from build123d import *

# Parameters (mm, degrees)
EXTRUDE_1_DEPTH     = 12
SKETCH_3_R          = 11
CUT_EXTRUDE_1_DEPTH = 111
SKETCH_4_R          = 12.5
CUT_EXTRUDE_2_DEPTH = 124.693168769
SKETCH_5_W          = 8
SKETCH_5_H          = 15.8
CUT_EXTRUDE_3_DEPTH = 124.693168769
SKETCH_6_R          = 3.4
CUT_EXTRUDE_4_DEPTH = 13
SKETCH_7_R          = 2.5
CUT_EXTRUDE_5_DEPTH = 10


with BuildPart() as part:
    # 草图1 → 旋转1 (revolve)
    with BuildSketch(Plane(origin=(0, 0, 0), x_dir=(1, 0, 0), z_dir=(0, 1, 0)), mode=Mode.PRIVATE) as revolve_1_sk:
        Polygon((0, 0), (25, 0), (25, -45), (40, -45), (40, -55), (0, -55), align=None)
    revolve(revolve_1_sk.sketch.rotate(Axis((0, 0, 0), (0, 0, 1)), 180), axis=Axis((0, 0, 0), (0, 0, 1)))

    # 草图2 → 凸台-拉伸1 (add)
    with BuildSketch(Plane(origin=(24, 0, 0), x_dir=(0, 0, -1), z_dir=(1, 0, 0))):
        with BuildLine():
            Line((-45, -20), (-90, -20))
            ThreePointArc((-90, -20), (-110, 0), (-90, 20))
            Line((-90, 20), (-45, 20))
            Line((-45, 20), (-45, -20))
        make_face()
    extrude_1 = extrude(amount=EXTRUDE_1_DEPTH)

    # 镜向1: 凸台-拉伸1 across plane
    add(extrude_1.mirror(Plane(origin=(0, 0, 0), x_dir=(0, 0, 1), z_dir=(1, 0, 0))))

    # 草图3 → 切除-拉伸1 (cut, symmetric)
    with BuildSketch(Plane(origin=(0, 0, 0), x_dir=(0, 0, -1), z_dir=(1, 0, 0))):
        with Locations((-90, 0)):
            Circle(SKETCH_3_R)
    extrude(amount=CUT_EXTRUDE_1_DEPTH, both=True, mode=Mode.SUBTRACT)

    # 草图4 → 切除-拉伸2 (cut, through all)
    with BuildSketch(Plane.XY):
        with Locations(Location((0, 0, 0), (0, 0, 180))):
            Circle(SKETCH_4_R)
    extrude(amount=CUT_EXTRUDE_2_DEPTH, mode=Mode.SUBTRACT)

    # 草图5 → 切除-拉伸3 (cut, through all)
    with BuildSketch(Plane.XY):
        with Locations((0, 7.9)):
            Rectangle(SKETCH_5_W, SKETCH_5_H)
    extrude(amount=CUT_EXTRUDE_3_DEPTH, mode=Mode.SUBTRACT)

    # 草图6 → 切除-拉伸4 (cut)
    with BuildSketch(Plane(origin=(0, 25, 0), x_dir=(1, 0, 0), z_dir=(0, 1, 0))):
        with Locations(Location((0, -20, 0), (0, 0, 270))):
            Circle(SKETCH_6_R)
    extrude(amount=-CUT_EXTRUDE_4_DEPTH, mode=Mode.SUBTRACT)

    # 草图7 → 切除-拉伸5 (cut)
    with BuildSketch(Plane(origin=(36, 0, 0), x_dir=(0, 0, -1), z_dir=(1, 0, 0))):
        with Locations((-90, 14.5)):
            Circle(SKETCH_7_R)
        with Locations((-90, -14.5)):
            Circle(SKETCH_7_R)
    cut_extrude_5 = extrude(amount=-CUT_EXTRUDE_5_DEPTH, mode=Mode.SUBTRACT)

    # 镜向2: 切除-拉伸5 across plane
    add(cut_extrude_5.mirror(Plane(origin=(0, 0, 0), x_dir=(0, 0, 1), z_dir=(1, 0, 0))), mode=Mode.SUBTRACT)


solid = part.part
Build history of the part. All positions in model axes, mm. A direction names the side the tool comes from. Give positions to 0.01 mm unless a question says otherwise; leave off trailing zeros. Order: outer loops, then holes, each group sorted by start corner. A loop starts at its lowest first (then second) coordinate and runs counter-clockwise, first axis right, second up. Notation, with made-up numbers: M 17,57.25 L 30,57.25 A17 ccw 30,87.25 Z; hole C -12,-8.75 d2. An arc over 180 degrees is marked long. Put each result on its own line as item: value.
Item 1: 3-axis set-ups, long thin cutter, end or side, ignore diameter. For faces 1 (the flat face through (-26, 15, 90)), 2 (the flat face through (-18.34, 17.22, 45)), 3 (the flat face through (24, 0, 76)): which of +Z, -Z, +X, -X, +Y, -Y reach the whole face in a straight line?
From the geometry:
face 1: -X
face 2: -Z
face 3: +Z, +Y, -Y
Item 2: Two-plate mould, pull along Z, no slides. Class faces 4 (the flat face through (-36, 0, 77)), 5 (the flat face through (-38, 0, 55)), 6 (the cylindrical face through (-30, 0, 101)): +Z half, -Z half, draft (parallel to the pull), parting line (faces both ways), or undercut.
From the geometry:
face 4: draft
face 5: +Z half
face 6: undercut
Item 3: Flat gauge pins, fed straight in: pin 1 Ø4.5 at (y, z) = (14.5, 90) entering from +X; pin 2 Ø4 at (x, z) = (-1, 34) entering from -Y; pin 3 Ø5.5 at (x, z) = (0, 20) entering from +Y. Where does each tip first touch, or does it go through?
From the geometry:
pin 1: stops at x = 26
pin 2: stops at y = -25
pin 3: stops at y = -12.19
Item 4: Probe line 1 (Y direction, x = -31.75, z = 90); line 2 (X direction, y = -0.5, z = 64); line 3 (Z direction, x = 0, y = 18.5). List the from-to ranges inside material, lowest first. Write a range as [from, to].
From the geometry:
line 1: y = [-20, -17], [-12, -11], [11, 12], [17, 20]
line 2: x = [-36, -24], [24, 36]
line 3: z = [0, 16.6], [23.4, 55]
Item 5: Slice it at D-D, the plane y = 14.5. Write the cut outline in (x, z), plus the area to 3 significant figures.
From the geometry:
outline: M -37.28,45 L -20.37,45 L -20.37,0 L -4,0 L -4,55 L -24,55 L -24,103.77 L -36,103.77 L -36,92.5 L -26,92.5 L -26,87.5 L -36,87.5 L -36,55 L -37.28,55 Z; M 4,0 L 20.37,0 L 20.37,45 L 37.28,45 L 37.28,55 L 36,55 L 36,87.5 L 26,87.5 L 26,92.5 L 36,92.5 L 36,103.77 L 24,103.77 L 24,55 L 4,55 Z
area: 3,210 mm2
Item 6: Slice it at B-B, the plane x = 32. Write the cut outline in (y, z), plus the area to 3 significant figures.
From the geometry:
outline: M -24,45 L 24,45 L 24,55 L 20,55 L 20,90 A20 ccw -20,90 L -20,55 L -24,55 Z; hole C -14.5,90 d5; hole C 0,90 d22; hole C 14.5,90 d5
area: 2,090 mm2
Item 7: Slice it at A-A, the plane z = 58.5. Write the cut outline in (x, y).
From the geometry:
outline: M -36,-20 L -24,-20 L -24,20 L -36,20 Z; M 24,-20 L 36,-20 L 36,20 L 24,20 Z
Item 8: Slice it at C-C, the plane z = 47. Write the cut outline in (x, y).
From the geometry:
outline: M -36,-20 L -34.64,-20 A40 ccw 34.64,-20 L 36,-20 L 36,-17.44 A40 ccw 36,17.44 L 36,20 L 34.64,20 A40 ccw -34.64,20 L -36,20 L -36,17.44 A40 ccw -36,-17.44 Z; hole M -4,11.84 A12.5 ccw long 4,11.84 L 4,15.8 L -4,15.8 Z
